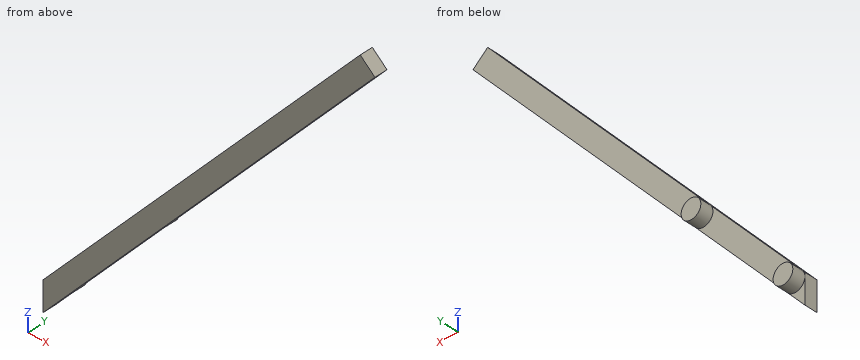
Autodesk Inventor part; units mm, degrees
ref_plane "YZ Plane" through (0, 0, 0) normal (1, 0, 0) x (0, 1, 0)
ref_plane "XZ Plane" through (0, 0, 0) normal (0, 1, 0) x (-1, 0, 0)
ref_plane "XY Plane" through (0, 0, 0) normal (0, 0, 1) x (1, 0, 0)
sketch "草圖1" plane through (0, 0, 0) normal (0, 1, 0) x (-1, 0, 0)
  line L0 (0, 0) -> (14.7102, 0)
  line L1 (14.7102, 0) -> (14.7102, -16.4216)
  line L2 (14.7102, -16.4216) -> (0, 0)
extrude "擠出1" add sketch "草圖1" along normal blind 1
sketch "草圖2" plane through (0, 1, 0) normal (0, 1, 0) x (1, 0, 0)
  circle A0 centre (-13.9602, 14.4603) radius 0.75
  line L0 (-14.7102, 16.4216) -> (-14.7102, 0)
  line L1 (0, 0) -> (-14.7102, 16.4216)
  dimension "d2" = 1.5
extrude "擠出2" add sketch "草圖2" along normal blind 1 contours A0
sketch "草圖4" plane through (0, 1, 0) normal (0, 1, 0) x (1, 0, 0)
  line L0 (-14.7102, 0) -> (0, 0)
  line L1 (-2.0138, 0) -> (-14.7102, 14.1735)
  line L2 (0, 0) -> (-13.4016, 14.9607)
  line L3 (-14.7102, 14.4603) -> (-14.7102, 0)
  point P0 (-1.1201, 1.2504)
  dimension "d7" = 1.5
extrude "擠出4" cut sketch "草圖4" against normal blind 10
sketch "草圖5" plane through (0, 1, 0) normal (0, 1, 0) x (1, 0, 0)
  circle A0 centre (-6.9543, 6.6393) radius 0.75
  line L0 (-14.5188, 13.9599) -> (-2.0138, 0)
  line L1 (0, 0) -> (-13.4016, 14.9607)
  circle A1 centre (-13.9602, 14.4603) radius 0.75
  dimension "d11" = 10.5
extrude "擠出5" add sketch "草圖5" along normal up to surface (1 mm away) contours A0
sketch "草圖6" plane through (0, 1, 0) normal (0, 1, 0) x (1, 0, 0)
  line L0 (-7.513, 6.1389) -> (-2.0138, 0)
  line L1 (0, 0) -> (-6.3957, 7.1398)
  line L2 (-2.0138, 0) -> (-0.8965, 1.0008)
  line L3 (-0.8965, 1.0008) -> (10.5719, -11.8019)
  line L4 (10.5719, -11.8019) -> (9.4546, -12.8027)
  line L5 (9.4546, -12.8027) -> (-2.0138, 0)
extrude "擠出6" add sketch "草圖6" against normal up to surface (1 mm away)
Here's how the part is built. I have some questions about the finished solid (model axes, mm). Coordinates: 2 decimals unless noted, no trailing zeros. Order: outer loops, then holes, each group sorted by start corner. A loop starts at its lowest first (then second) coordinate and runs counter-clockwise, first axis right, second up.
Item 1: If we section it at C-C on z = 8.5: List the corners of the cut face in (x, y) for me.
Result sheet:
outline: (5.6, 0) - (7.61, 0) - (7.61, 1) - (5.6, 1) - close
Item 2: If we section it at A-A on y = 0.35: List the corners of the cut face in (x, z) for me, plus the area to 3 significant figures.
Result sheet:
outline: (-14.71, -16.42) - (0, 0) - (10.57, 11.8) - (9.45, 12.8) - (-2.01, 0) - (-14.71, -14.17) - close
area: 55.6 mm2
Item 3: I need wall thicknesses on line 1 (Y direction, x = -9, z = -8.5); line 2 (X direction, y = 0.25, z = 3.75); line 3 (X direction, y = 0.5, z = 6.5). Which ranges of each line are inside material? Lowest first, please.
Result sheet:
line 1: y = 0 to 1
line 2: x = 1.35 to 3.36
line 3: x = 3.81 to 5.82
Item 4: If we section it at B-B on x = 5: List the corners of the cut face in (y, z) for me, plus the area to 3 significant figures.
Result sheet:
outline: (0, 5.58) - (1, 5.58) - (1, 7.83) - (0, 7.83) - close
area: 2.25 mm2
Item 5: For P1, Ø9, axis at x = 0.5, z = -1.5, coming from the +Y side, with a flat end and sliding along its axis, tell me the tip position at first contact or that it passes through.
Result sheet:
P1: stops at y = 1
